Geometry: final body of the model. Coordinates: model frame, mm. A direction names the side the tool comes from. Round coordinates to 2 decimals unless told otherwise and drop trailing zeros. Write each loop counter-clockwise with the first axis right and the second up, starting at its lowest first coordinate (ties: lowest second). Pieces come first, ordered by that corner, then holes. Notation, with made-up numbers: (31, 20) - (87, 20) arc R9 ccw to (87, 28) - close; hole circle Ø1 at (-38, 45.5). An arc over 180 degrees is marked (long way). Write each question's results on one line, items separated by ' | '.
from build123d import *

# Parameters (mm, degrees)
F0_W      = 1200
F0_H      = 700
F1_DEPTH  = 700
F3_DEPTH  = 700.001
F4_R      = 150
F5_DEPTH  = 700.001
F6_W      = 260
F6_H      = 398.8438928255
F7_DEPTH  = 300.001
F8_W      = 260
F8_H      = 102.9841262038
F9_DEPTH  = 300.001
F10_W     = 359.9333584309
F10_H     = 237.0417833328
F11_DEPTH = 1200.001


with BuildPart() as f1:
    # F0 (on Front) → F1 (new body)
    with BuildSketch(Plane.XZ):
        Rectangle(F0_W, F0_H)
    extrude(amount=F1_DEPTH)

    # F2 (on face) → F3 (cut, through all)
    with BuildSketch(Plane.XZ.offset(700)):
        with BuildLine():
            Line((-600, -50), (17.1572875254, -50))
            ThreePointArc((17.1572875254, -50), (55.0510257217, 223.2050807569), (300, 350))
            Line((300, 350), (-600, 350))
            Line((-600, 350), (-600, -50))
        make_face()
        with BuildLine():
            ThreePointArc((300, 350), (512.132034356, 262.132034356), (600, 50))
            Line((600, 50), (600, 350))
            Line((600, 350), (300, 350))
        make_face()
    extrude(amount=-F3_DEPTH, mode=Mode.SUBTRACT)

    # F4 (on face) → F5 (cut, through all)
    with BuildSketch(Plane.XZ.offset(700)):
        with Locations((300, 50)):
            Circle(F4_R)
    extrude(amount=-F5_DEPTH, mode=Mode.SUBTRACT)

    # F6 (on face) → F7 (cut, through all)
    with BuildSketch(Plane.XY.offset(-50)):
        with Locations((-362.4188005924, -305.1174879074)):
            Rectangle(F6_W, F6_H)
    extrude(amount=-F7_DEPTH, mode=Mode.SUBTRACT)

    # F8 (on face) → F9 (cut, through all)
    with BuildSketch(Plane.XY.offset(-50)):
        with Locations((-362.4188005924, -556.0314974221)):
            Rectangle(F8_W, F8_H)
    extrude(amount=-F9_DEPTH, mode=Mode.SUBTRACT)

    # F10 (on face) → F11 (cut, through all)
    with BuildSketch(Plane(origin=(-600, 0, 0), x_dir=(0, -1, 0), z_dir=(-1, 0, 0))):
        with Locations((350, -350)):
            Rectangle(F10_W, F10_H)
    extrude(amount=-F11_DEPTH, mode=Mode.SUBTRACT)


solid = f1.part
Q1. Access query for faces 4 (the flat face through (-547, -529.967, -292)), 5 (the flat face through (600, -345, -108)), 6 (the flat face through (-364, -105.696, -198)). Directions: +Z, -Z, +X, -X, +Y, -Y. A direction counts if a zero-diameter tool reaches every point of the face in a straight line with its end or side. Return the directions, or none.
Answer block:
face 4: -Z, +X, -X | face 5: +Z, -Z, +X, +Y, -Y | face 6: +Z, -Z
Q2. Pin query (flat end, axial travel): pin 1 (12 mm diameter, centred on x = 166.5, y = -504, fed in from -Z); pin 2 (5 mm diameter, centred on y = -369, z = 274, fed in from -X); pin 3 (4 mm diameter, centred on y = -145, z = 155.5, fed in from -X). Return the tip coordinate at first contact, or that it passes through.
Answer block:
pin 1: z = -231.48 | pin 2: x = 97.67 | pin 3: x = 18.42
Q3. Mould query, pull axis Y, two halves, no side actions, for faces 1 (the cylindrical face through (242.079, -354.9, 344.356)), 2 (the flat face through (125, 0, -73)), 3 (the flat face through (-547, -347, -231.479)). Classes: pulls with the +Y half, pulls with the -Y half, needs draft (parallel to the pull), parting line crosses it, or undercut.
Answer block:
face 1: needs draft | face 2: pulls with the +Y half | face 3: undercut
Q4. Ray query, line 1 along Z through (x, y) = (300, -249); line 2 along X through (y, z) = (-123, -152.5); line 3 along Y through (x, z) = (-367, -169). Return the intervals inside material, ascending.
Answer block:
line 1: -231.48 to -100, 200 to 350 | line 2: -600 to -492.42, -232.42 to 600 | line 3: -700 to -607.52, -105.7 to 0
Q5. Section query C-C, the plane x = -346. Return loops of the section in (y, z), plus the area to 3 significant figures.
Answer block:
outline: (-700, -350) - (-607.52, -350) - (-607.52, -50) - (-700, -50) - close; (-105.7, -350) - (0, -350) - (0, -50) - (-105.7, -50) - close | area: 59,500 mm2
Q6. Section query D-D, the plane y = -127.5. Return loops of the section in (x, z).
Answer block:
outline: (-600, -350) - (-492.42, -350) - (-492.42, -50) - (-600, -50) - close; (-232.42, -350) - (600, -350) - (600, 50) arc R300 ccw (long way) to (17.16, -50) - (-232.42, -50) - close; hole circle Ø300 at (300, 50)
Q7. Section query A-A, the plane y = -422.5. Return loops of the section in (x, z), plus the area to 3 significant figures.
Answer block:
outline: (-600, -231.48) - (-492.42, -231.48) - (-492.42, -50) - (-600, -50) - close; (-232.42, -231.48) - (600, -231.48) - (600, 50) arc R300 ccw (long way) to (17.16, -50) - (-232.42, -50) - close; hole circle Ø300 at (300, 50) | area: 301,000 mm2
Q8. Section query B-B, the plane z = -297. Return loops of the section in (x, y), plus the area to 3 significant figures.
Answer block:
outline: (-600, -700) - (600, -700) - (600, -529.97) - (-232.42, -529.97) - (-232.42, -607.52) - (-492.42, -607.52) - (-492.42, -529.97) - (-600, -529.97) - close; (-600, -170.03) - (-492.42, -170.03) - (-492.42, -105.7) - (-232.42, -105.7) - (-232.42, -170.03) - (600, -170.03) - (600, 0) - (-600, 0) - close | area: 371,000 mm2
